from build123d import *

# Parameters (mm, degrees)
F2_SIZE  = 0.79375
F3_R     = 7.9375
F4_DEPTH = 25.4
F5_R     = 1.5875
F7_D     = 3.4544
F8_D     = 6.5278
F8_DEPTH = 12.954
F8_TIP   = 1.9611489744


with BuildPart() as f1:
    # F0 (on Front) → F1 (revolve)
    with BuildSketch(Plane.XZ):
        Polygon((-11.1125, 0), (0, 0), (0, 11.3848719395), (-6.0776280605, 17.4625), (-11.1125, 17.4625), align=None)
    revolve(axis=Axis((0, 0, 5.6924359697), (0, 0, 1)))

    # F2
    f2_edges = [f1.edges().sort_by_distance(p)[0] for p in [
        (11.1125, 0, 0),
        (11.1125, 0, 17.4625),
    ]]
    chamfer(f2_edges, length=F2_SIZE)

    # F3 (on Front) → F4 (cut)
    with BuildSketch(Plane.XZ):
        with Locations((0, 23.5401280605)):
            Circle(F3_R)
    extrude(amount=F4_DEPTH, mode=Mode.SUBTRACT)

    # F5
    f5_edges = [f1.edges().sort_by_distance(p)[0] for p in [
        (0, -4.217756, 15.602628),
    ]]
    fillet(f5_edges, radius=F5_R)

    # F7 (through all)
    with Locations(Plane(origin=(0, 0, 0), x_dir=(1, 0, 0), z_dir=(0, 0, -1))):
        with Locations((0, 0)):
            Hole(F7_D / 2)

    # F8
    with Locations(Plane(origin=(0, 0, 0), x_dir=(1, 0, 0), z_dir=(0, 0, -1))):
        with Locations((6.35, 0), (-6.35, 0)):
            Hole(F8_D / 2, depth=F8_DEPTH)
            with Locations((0, 0, -(F8_DEPTH + F8_TIP / 2))):  # 118° drill point
                Cone(0, F8_D / 2, F8_TIP, mode=Mode.SUBTRACT)


solid = f1.part
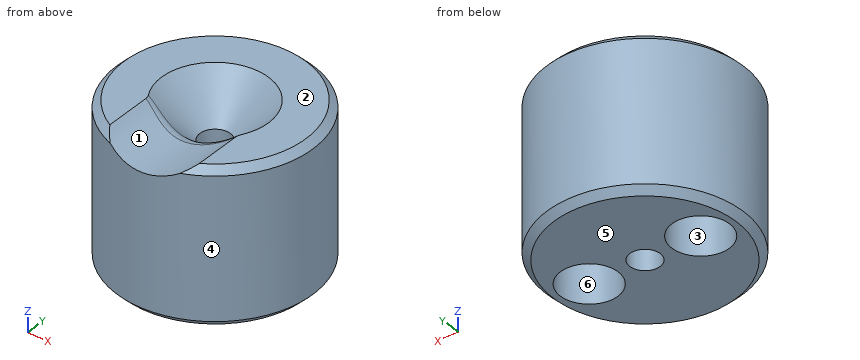
Model file for the job. Use its own axes, mm. Face numbers are marked on the shaded views. A direction names the side the tool comes from. Coordinates: 2 decimals unless noted, no trailing zeros. Write each question's results on one line, items separated by ' | '. Start each with the question number.
1) Mould opens along X. For the marked faces 4, 5 and 6 say: pulls with the +X half, pulls with the -X half, needs draft (parallel to the pull), parting line crosses it, or undercut.
2) 3-axis set-ups, long thin cutter, end or side, ignore diameter. For the marked faces 1, 2 and 3: which of +Z, -Z, +X, -X, +Y, -Y reach the whole face in a straight line?
3) Probe line 1 along Y through (x, z) = (0, 10.25); line 2 along X through (y, z) = (0.75, 4.5); line 3 along Y through (x, z) = (-6.35, 6.25). List the from-to ranges inside material, lowest first. Write a range as from..to.
4) Flat gauge pins, fed straight in: P1, Ø6, axis at x = 3.5, z = 10.5, coming from the -Y side; P2, Ø6, axis at x = -6.35, y = 0, coming from the -Z side; P3, Ø1, axis at x = 6.5, z = 4, coming from the -Y side. Where does each tip first touch, or does it go through?
5) Cut at A-A (z = 4.25). Count the separate pieces of the cut face and the enclosed holes in it, then the cut area to 3 significant figures.
Returned:
1) face 4: parting line crosses it | face 5: needs draft | face 6: undercut
2) face 1: +Z, -Y | face 2: +Z, +X, -X, +Y, -Y | face 3: -Z
3) line 1: -11.11..-1.73, 1.73..11.11 | line 2: -11.09..-9.53, -3.17..-1.56, 1.56..3.17, 9.53..11.09 | line 3: -9.12..-3.26, 3.26..9.12
4) P1: y = -11.1 | P2: z = 13.11 | P3: y = -9.35
5) separate pieces: 1 | enclosed holes: 3 | area: 312 mm^2
